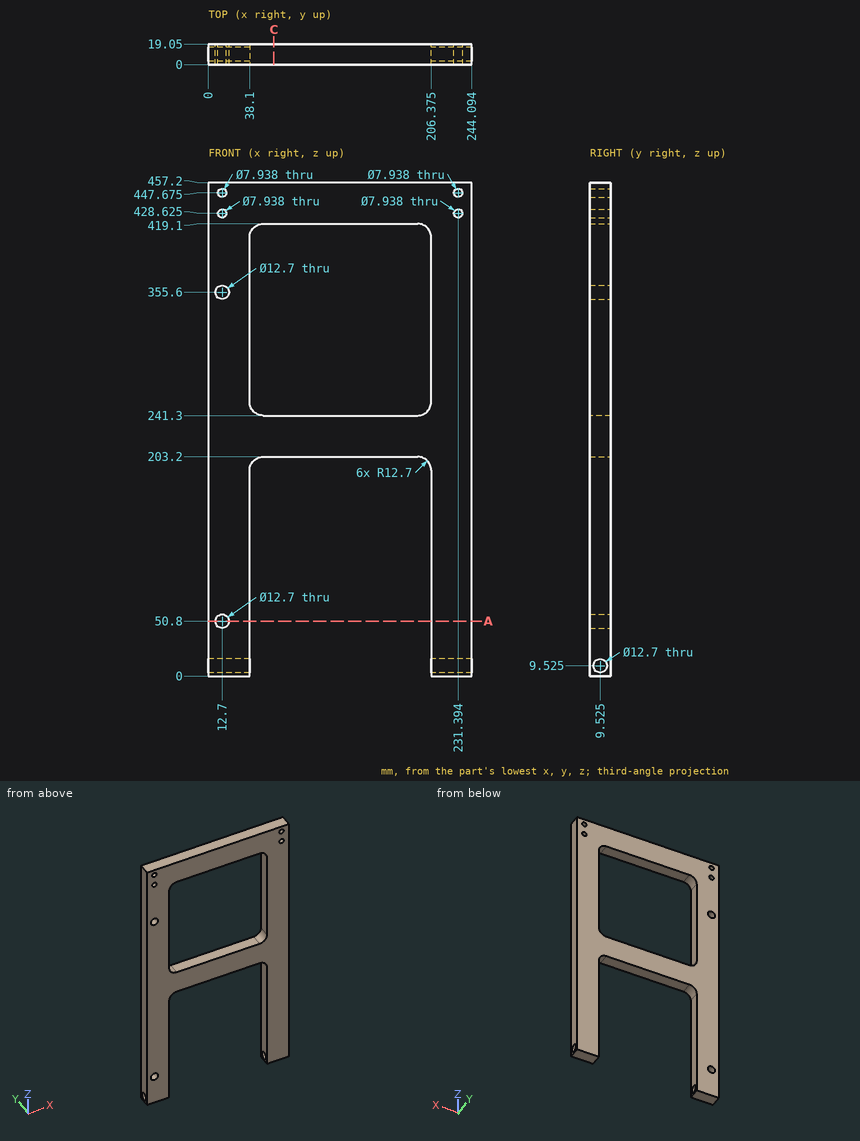
Geometry check sheet. Reference: drawing and pictorial views, mm from the part's lowest x, y, z. Round coordinates to 2 decimals unless told otherwise and drop trailing zeros. Loops run counter-clockwise (first coordinate to the right, second up) from the corner with the lowest first, then second, coordinate; pieces in that order, holes last. Notation, with made-up numbers: M 4.25,20 L 44.25,20 A20 cw 44.25,26 Z; hole C 19.5,25.25 d2. An arc over 180 degrees is marked long. Return JSON: item names as keys, results as strings. Group by question number.
(1) Scan lines: line 1 along X through (y, z) = (6, 120) (1 decimal); line 2 along Z through (x, y) = (161.5, 3.75); line 3 along Z through (x, y) = (17, 5.75) (1 decimal). Record each from-to range of solid material in increasing order. Write a range as [from, to].
(2) Section check C-C, the plane x = 60.5. Enter the section's corners in (y, z).
(3) Go/stop test with flat-tipped pins: pin 1 (9.5 mm diameter, centred on x = 91, y = 13.5, fed in from -Z); pin 2 (9.5 mm diameter, centred on y = 9, z = 335, fed in from -X); pin 3 (4 mm diameter, centred on x = 46.5, y = 12, fed in from -Z). Record where each tip stops, or that it passes through.
(4) Section check A-A, the plane z = 50.8. Give the number of separate pieces and of enclosed holes in the cut face, and give its area (3 significant figures).
Data:
{
 "1": {"line 1": "[0, 38.1], [206.4, 244.1]", "line 2": "[203.2, 241.3], [419.1, 457.2]", "line 3": "[0, 4.4], [14.6, 46.1], [55.5, 350.9], [360.3, 457.2]"},
 "2": {"outline": "M 0,203.2 L 19.05,203.2 L 19.05,241.3 L 0,241.3 Z; M 0,419.1 L 19.05,419.1 L 19.05,457.2 L 0,457.2 Z"},
 "3": {"pin 1": "z = 203.2", "pin 2": "x = 0", "pin 3": "z = 201.53"},
 "4": {"separate pieces": "3", "enclosed holes": "0", "area": "1,200 mm²"}
}
